Geometry check sheet. Reference: drawing and pictorial views, mm from the part's lowest x, y, z. Give positions to 0.01 mm unless a question says otherwise; leave off trailing zeros. Write each loop counter-clockwise with the first axis right and the second up, starting at its lowest first coordinate (ties: lowest second). Pieces come first, ordered by that corner, then holes. Notation, with made-up numbers: M 38.25,61 L 43.25,61 A27 cw 43.25,81 Z; hole C -27.75,13.5 d4. An arc over 180 degrees is marked long. One line per item, written item: value. Start each with the question number.
1. Cross-section at A-A on x = 11. Record the cut outline in (y, z).
2. Cross-section at C-C on x = 23. Record the cut outline in (y, z).
3. Gauge pin test, flat end, axial feed: pin 1 (4.5 mm diameter, centred on x = 24.125, y = 24.125, fed in from -Z). Record the tip position at first contact, or that the pin passes through.
4. Release check for a two-part mould opening along X. For the marked faces 1, 2 and 3 record: pulls with the +X half, pulls with the -X half, needs draft (parallel to the pull), parting line crosses it, or undercut.
5. Cross-section at D-D on z = 2.6. Record the cut outline in (x, y) (3 decimals), then the cut area to 3 significant figures.
6. Cross-section at B-B on y = 37.5. Record the cut outline in (x, z).
7. Scan lines: line 1 (X direction, y = 37, z = 2.45); line 2 (Y direction, x = 38, z = 1.8); line 3 (X direction, y = 36, z = 1.3). Record each from-to range of solid material in increasing order.
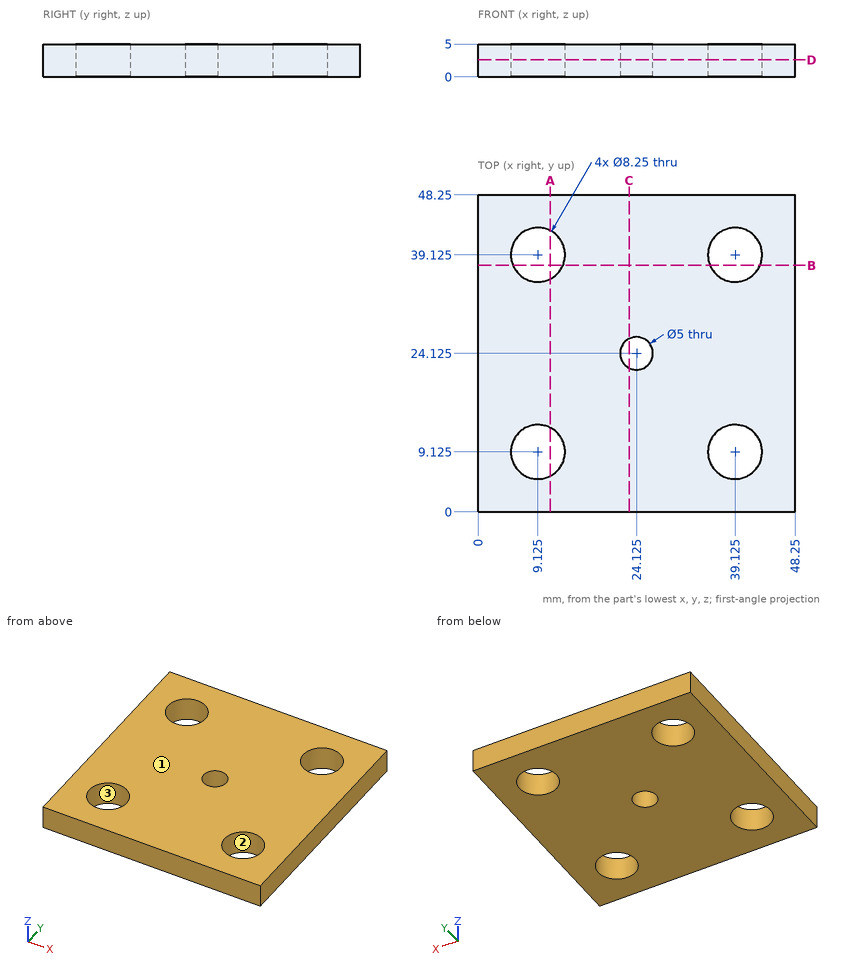
Report:
1. outline: M 0,0 L 5.45,0 L 5.45,5 L 0,5 Z; M 12.8,0 L 35.45,0 L 35.45,5 L 12.8,5 Z; M 42.8,0 L 48.25,0 L 48.25,5 L 42.8,5 Z
2. outline: M 0,0 L 21.89,0 L 21.89,5 L 0,5 Z; M 26.36,0 L 48.25,0 L 48.25,5 L 26.36,5 Z
3. pin 1: passes through
4. face 1: needs draft
4. face 2: undercut
4. face 3: undercut
5. outline: M 0,0 L 48.25,0 L 48.25,48.25 L 0,48.25 Z; hole C 9.125,9.125 d8.25; hole C 9.125,39.125 d8.25; hole C 24.125,24.125 d5; hole C 39.125,9.125 d8.25; hole C 39.125,39.125 d8.25
5. area: 2,090 mm^2
6. outline: M 0,0 L 5.33,0 L 5.33,5 L 0,5 Z; M 12.92,0 L 35.33,0 L 35.33,5 L 12.92,5 Z; M 42.92,0 L 48.25,0 L 48.25,5 L 42.92,5 Z
7. line 1: x = 0 to 5.59, 12.66 to 35.59, 42.66 to 48.25
7. line 2: y = 0 to 5.16, 13.09 to 35.16, 43.09 to 48.25
7. line 3: x = 0 to 6.43, 11.82 to 36.43, 41.82 to 48.25
